The listing builds one solid part. Answer for the finished solid, in the listing's coordinates (mm). A direction names the side the tool comes from. Coordinates: 2 decimals unless noted, no trailing zeros. Loops run counter-clockwise (first coordinate to the right, second up) from the corner with the lowest first, then second, coordinate; pieces in that order, holes last. Notation, with made-up numbers: (-16.75, 80) - (42.25, 80) arc R13 cw to (42.25, 101) - close; hole circle Ø9 at (-33, 10). An arc over 180 degrees is marked (long way). Write each question's results on one line, items separated by ' | '. Start each with the question number.
(1) Find section D-D on y = 16. Determine the outline of the cut face in (x, z).
(2) Find section B-B on x = 0. Determine the outline of the cut face in (y, z), then the cut area to 3 significant figures.
(3) For faces 1 (the flat face through (32.1, -16, 20)), 2 (the flat face through (-32.1, -16, 20)), 3 (the flat face through (49.389, -36, 20)), determine the directions among +Z, -Z, +X, -X, +Y, -Y from which every point of the face is accessible in a straight line to the end or side of a thin tool.
(4) Given pin 1 Ø12.5 at (x, z) = (-35.5, 14) entering from +Y; pin 2 Ø1.5 at (y, z) = (-24, 17.5) entering from -X; pin 3 Ø1.5 at (x, z) = (10.5, 23.5) entering from +Y, each flat-ended and moving along its own axis, determine where each tip first touches the part or whether it passes through.
(5) Consider line 1 (X direction, y = -34.5, z = 35); line 2 (X direction, y = -1, z = 27); line 3 (X direction, y = -32, z = 26). Determine where each line is inside the solid, lowest interval first. Write a range as from..to.
(6) Find section A-A on z = 5. Determine the outline of the cut face in (x, y).
(7) Find section C-C on y = -33.5. Determine the outline of the cut face in (x, z), then the cut area to 3 significant figures.
(8) Determine the mould class of faces 4 (the cylindrical face through (40.785, -36.156, 37.883)), 5 (the cylindrical face through (0.706, 32.092, 19.72)), 6 (the flat face through (3, -28, 40)), 7 (the cylindrical face through (39.28, -36.16, 6.24)) for opening direction Z: released by +Z, released by -Z, zero draft, split by the parting line, or undercut.
from build123d import *

# Parameters (mm, degrees)
SKETCH_1_R              = 26.1
EXTRUDE_1_DEPTH         = 40
HOLE_WIZARD_6_5_6_5_1_D = 6.5


with BuildPart() as part:
    # 草图1 → 凸台-拉伸1 (new body)
    with BuildSketch(Plane.XY):
        with BuildLine():
            Line((-32.1, 0), (-32.1, -32.1))
            Line((-32.1, -32.1), (-43.611358786, -32.1))
            Line((-43.611358786, -32.1), (-43.611358786, -40.1))
            Line((-43.611358786, -40.1), (49.388641214, -40.1))
            Line((49.388641214, -40.1), (49.388641214, -32.1))
            Line((49.388641214, -32.1), (32.1, -32.1))
            Line((32.1, -32.1), (32.1, 0))
            ThreePointArc((32.1, 0), (0, 32.1), (-32.1, 0))
        make_face()
        Circle(SKETCH_1_R, mode=Mode.SUBTRACT)
    extrude(amount=EXTRUDE_1_DEPTH)

    # Ø6.5 (6.5) 直径孔1 (through all)
    with Locations(Plane(origin=(0, -32.1, 0), x_dir=(1, 0, 0), z_dir=(0, 1, 0))):
        with Locations((42.285158123, -5), (42.285158123, -35), (-36.314841877, -35), (-36.314841877, -5)):
            Hole(HOLE_WIZARD_6_5_6_5_1_D / 2)


solid = part.part
Values:
1) outline: (-27.83, 0) - (-20.62, 0) - (-20.62, 40) - (-27.83, 40) - close; (20.62, 0) - (27.83, 0) - (27.83, 40) - (20.62, 40) - close
2) outline: (-40.1, 0) - (-26.1, 0) - (-26.1, 40) - (-40.1, 40) - close; (26.1, 0) - (32.1, 0) - (32.1, 40) - (26.1, 40) - close | area: 800 mm²
3) face 1: +Z, -Z, +X, +Y | face 2: +Z, -Z, -X, +Y | face 3: +Z, -Z, +X, +Y, -Y
4) pin 1: stops at y = 13.22 | pin 2: stops at x = -32.1 | pin 3: stops at y = 30.58
5) line 1: x = -43.61..-39.56, -33.06..39.04, 45.54..49.39 | line 2: x = -32.1..-26.08, 26.08..32.1 | line 3: x = -32.1..32.1
6) outline: (-43.61, -40.1) - (-39.56, -40.1) - (-39.56, -32.1) - (-43.61, -32.1) - close; (-33.06, -40.1) - (39.04, -40.1) - (39.04, -32.1) - (32.1, -32.1) - (32.1, 0) arc R32.1 ccw to (-32.1, 0) - (-32.1, -32.1) - (-33.06, -32.1) - close; (45.54, -40.1) - (49.39, -40.1) - (49.39, -32.1) - (45.54, -32.1) - close; hole circle Ø52.2 at (0, 0)
7) outline: (-43.61, 0) - (49.39, 0) - (49.39, 40) - (-43.61, 40) - close; hole circle Ø6.5 at (-36.31, 5); hole circle Ø6.5 at (-36.31, 35); hole circle Ø6.5 at (42.29, 5); hole circle Ø6.5 at (42.29, 35) | area: 3,590 mm²
8) face 4: undercut | face 5: zero draft | face 6: released by +Z | face 7: undercut
